```python
from build123d import *

# Parameters (mm, degrees)
BOSS_EXTRUDE1_DEPTH = 4
SKETCH2_R           = 1.6
CUT_EXTRUDE1_DEPTH  = 80.797158741
CUT_EXTRUDE2_DEPTH  = 2
CUT_EXTRUDE3_DEPTH  = 1.5
SKETCH5_R           = 4
BOSS_EXTRUDE3_DEPTH = 2
SKETCH6_R           = 1.5
CUT_EXTRUDE4_DEPTH  = 80.797158741
FILLET1_R           = 3


with BuildPart() as part:
    # Sketch1 → Boss-Extrude1 (new body)
    with BuildSketch(Plane(origin=(0, 0, 0), x_dir=(1, 0, 0), z_dir=(0, 1, 0))):
        Polygon((-12.5, 0), (12.5, 0), (23.338026386, 1.062677778), (36.065948447, -11.665244283), (35.003270669, -22.503270669), (35.003270669, -47.503270669), (36.065948447, -58.341297055), (23.338026386, -71.069219116), (12.5, -70.006541338), (-12.5, -70.006541338), (-23.338026386, -71.069219116), (-36.065948447, -58.341297055), (-35.003270669, -47.503270669), (-35.003270669, -22.503270669), (-36.065948447, -11.665244283), (-23.338026386, 1.062677778), align=None)
    extrude(amount=BOSS_EXTRUDE1_DEPTH)

    # Sketch2 → Cut-Extrude1 (cut, through all)
    with BuildSketch(Plane(origin=(0, 4, 0), x_dir=(1, 0, 0), z_dir=(0, 1, 0))):
        with Locations(Location((22.63, -3.893270669, 0), (0, 0, 270))):
            Circle(SKETCH2_R)
        with Locations(Location((31.11, -12.373270669, 0), (0, 0, 270))):
            Circle(SKETCH2_R)
        with Locations(Location((-31.11, -12.373270669, 0), (0, 0, 90))):
            Circle(SKETCH2_R)
        with Locations(Location((-22.63, -3.893270669, 0), (0, 0, 90))):
            Circle(SKETCH2_R)
        with Locations(Location((31.11, -57.633270669, 0), (0, 0, 90))):
            Circle(SKETCH2_R)
        with Locations(Location((22.63, -66.113270669, 0), (0, 0, 90))):
            Circle(SKETCH2_R)
        with Locations(Location((-22.63, -66.113270669, 0), (0, 0, 270))):
            Circle(SKETCH2_R)
        with Locations(Location((-31.11, -57.633270669, 0), (0, 0, 270))):
            Circle(SKETCH2_R)
    extrude(amount=-CUT_EXTRUDE1_DEPTH, mode=Mode.SUBTRACT)

    # Sketch3 → Cut-Extrude2 (cut)
    with BuildSketch(Plane(origin=(0, 4, 0), x_dir=(1, 0, 0), z_dir=(0, 1, 0))):
        Polygon((-17.672782103, -6), (17.672782103, -6), (29.003270669, -17.330488566), (29.003270669, -52.676052772), (17.672782103, -64.006541338), (-17.672782103, -64.006541338), (-29.003270669, -52.676052772), (-29.003270669, -17.330488566), align=None)
    extrude(amount=-CUT_EXTRUDE2_DEPTH, mode=Mode.SUBTRACT)

    # Sketch4 → Cut-Extrude3 (cut)
    with BuildSketch(Plane(origin=(0, 2, 0), x_dir=(1, 0, 0), z_dir=(0, 1, 0))):
        with BuildLine():
            Line((-4.595346553, -50.006541338), (4.595346553, -50.006541338))
            ThreePointArc((4.595346553, -50.006541338), (5.867462624, -50.289609115), (6.899515315, -51.085394202))
            Line((6.899515315, -51.085394202), (13.569676517, -59.085394202))
            ThreePointArc((13.569676517, -59.085394202), (13.982439977, -62.278657408), (11.265507754, -64.006541338))
            Line((11.265507754, -64.006541338), (-11.265507754, -64.006541338))
            ThreePointArc((-11.265507754, -64.006541338), (-13.982439977, -62.278657408), (-13.569676517, -59.085394202))
            Line((-13.569676517, -59.085394202), (-6.899515315, -51.085394202))
            ThreePointArc((-6.899515315, -51.085394202), (-5.867462624, -50.289609115), (-4.595346553, -50.006541338))
        make_face()
        with BuildLine():
            Line((-24.082123534, -48.572947186), (-16.082123534, -41.902785984))
            ThreePointArc((-16.082123534, -41.902785984), (-15.286338446, -40.870733292), (-15.003270669, -39.598617222))
            Line((-15.003270669, -39.598617222), (-15.003270669, -30.407924116))
            ThreePointArc((-15.003270669, -30.407924116), (-15.286338446, -29.135808045), (-16.082123534, -28.103755354))
            Line((-16.082123534, -28.103755354), (-24.082123534, -21.433594152))
            ThreePointArc((-24.082123534, -21.433594152), (-27.27538674, -21.020830692), (-29.003270669, -23.737762914))
            Line((-29.003270669, -23.737762914), (-29.003270669, -46.268778423))
            ThreePointArc((-29.003270669, -46.268778423), (-27.27538674, -48.985710646), (-24.082123534, -48.572947186))
        make_face()
        with BuildLine():
            Line((-13.569676517, -10.921147135), (-6.899515315, -18.921147135))
            ThreePointArc((-6.899515315, -18.921147135), (-5.867462624, -19.716932223), (-4.595346553, -20))
            Line((-4.595346553, -20), (4.595346553, -20))
            ThreePointArc((4.595346553, -20), (5.867462624, -19.716932223), (6.899515315, -18.921147135))
            Line((6.899515315, -18.921147135), (13.569676517, -10.921147135))
            ThreePointArc((13.569676517, -10.921147135), (13.982439977, -7.727883929), (11.265507754, -6))
            Line((11.265507754, -6), (-11.265507754, -6))
            ThreePointArc((-11.265507754, -6), (-13.982439977, -7.727883929), (-13.569676517, -10.921147135))
        make_face()
        with BuildLine():
            Line((24.082123534, -21.433594152), (16.082123534, -28.103755354))
            ThreePointArc((16.082123534, -28.103755354), (15.286338446, -29.135808045), (15.003270669, -30.407924116))
            Line((15.003270669, -30.407924116), (15.003270669, -39.598617222))
            ThreePointArc((15.003270669, -39.598617222), (15.286338446, -40.870733292), (16.082123534, -41.902785984))
            Line((16.082123534, -41.902785984), (24.082123534, -48.572947186))
            ThreePointArc((24.082123534, -48.572947186), (27.27538674, -48.985710646), (29.003270669, -46.268778423))
            Line((29.003270669, -46.268778423), (29.003270669, -23.737762914))
            ThreePointArc((29.003270669, -23.737762914), (27.27538674, -21.020830692), (24.082123534, -21.433594152))
        make_face()
    extrude(amount=-CUT_EXTRUDE3_DEPTH, mode=Mode.SUBTRACT)

    # Sketch5 → Boss-Extrude3 (add)
    with BuildSketch(Plane(origin=(0, 2, 0), x_dir=(1, 0, 0), z_dir=(0, 1, 0))):
        with Locations(Location((15.25, -19.753270669, 0), (0, 0, 90))):
            Circle(SKETCH5_R)
        with Locations(Location((-15.25, -19.753270669, 0), (0, 0, 90))):
            Circle(SKETCH5_R)
        with Locations(Location((-15.25, -50.253270669, 0), (0, 0, 90))):
            Circle(SKETCH5_R)
        with Locations(Location((15.25, -50.253270669, 0), (0, 0, 90))):
            Circle(SKETCH5_R)
    extrude(amount=BOSS_EXTRUDE3_DEPTH)

    # Sketch6 → Cut-Extrude4 (cut, through all)
    with BuildSketch(Plane(origin=(0, 4, 0), x_dir=(1, 0, 0), z_dir=(0, 1, 0))):
        with Locations(Location((15.25, -19.753270669, 0), (0, 0, 270))):
            Circle(SKETCH6_R)
        with Locations(Location((15.25, -50.253270669, 0), (0, 0, 270))):
            Circle(SKETCH6_R)
        with Locations(Location((-15.25, -50.253270669, 0), (0, 0, 270))):
            Circle(SKETCH6_R)
        with Locations(Location((-15.25, -19.753270669, 0), (0, 0, 270))):
            Circle(SKETCH6_R)
    extrude(amount=-CUT_EXTRUDE4_DEPTH, mode=Mode.SUBTRACT)

    # Fillet1
    # the kernel refuses this fillet: 3 mm, written as the material it adds along each edge
    with BuildSketch(Plane(origin=(15.25, 2, 19.753270669), x_dir=(0, 0, -1), z_dir=(1, 0, 0))) as fillet1_piece_1:
        with BuildLine():
            CenterArc((6.828427125, 3), FILLET1_R, 199.471220634, 70.528779366)
            Line((4, 2), (3.943431458, 1.98))
            ThreePointArc((3.943431458, 1.98), (3.94, 1), (3.94, 0))
            Line((3.94, 0), (4, -0.06))
            Line((4, -0.06), (6.828427125, -0.06))
            Line((6.828427125, -0.06), (6.828427125, 0))
        make_face()
    revolve(axis=Axis((15.25, 2, 19.753270669), (0, 1, 0)))
    with BuildSketch(Plane(origin=(-15.25, 2, 19.753270669), x_dir=(0, 0, -1), z_dir=(1, 0, 0))) as fillet1_piece_2:
        with BuildLine():
            CenterArc((6.828427125, 3), FILLET1_R, 199.471220634, 70.528779366)
            Line((4, 2), (3.943431458, 1.98))
            ThreePointArc((3.943431458, 1.98), (3.94, 1), (3.94, 0))
            Line((3.94, 0), (4, -0.06))
            Line((4, -0.06), (6.828427125, -0.06))
            Line((6.828427125, -0.06), (6.828427125, 0))
        make_face()
    revolve(axis=Axis((-15.25, 2, 19.753270669), (0, 1, 0)))
    with BuildSketch(Plane(origin=(-15.25, 2, 50.253270669), x_dir=(0, 0, -1), z_dir=(1, 0, 0))) as fillet1_piece_3:
        with BuildLine():
            CenterArc((6.828427125, 3), FILLET1_R, 199.471220634, 70.528779366)
            Line((4, 2), (3.943431458, 1.98))
            ThreePointArc((3.943431458, 1.98), (3.94, 1), (3.94, 0))
            Line((3.94, 0), (4, -0.06))
            Line((4, -0.06), (6.828427125, -0.06))
            Line((6.828427125, -0.06), (6.828427125, 0))
        make_face()
    revolve(axis=Axis((-15.25, 2, 50.253270669), (0, 1, 0)))
    with BuildSketch(Plane(origin=(15.25, 2, 50.253270669), x_dir=(0, 0, -1), z_dir=(1, 0, 0))) as fillet1_piece_4:
        with BuildLine():
            CenterArc((6.828427125, 3), FILLET1_R, 199.471220634, 70.528779366)
            Line((4, 2), (3.943431458, 1.98))
            ThreePointArc((3.943431458, 1.98), (3.94, 1), (3.94, 0))
            Line((3.94, 0), (4, -0.06))
            Line((4, -0.06), (6.828427125, -0.06))
            Line((6.828427125, -0.06), (6.828427125, 0))
        make_face()
    revolve(axis=Axis((15.25, 2, 50.253270669), (0, 1, 0)))


solid = part.part
```
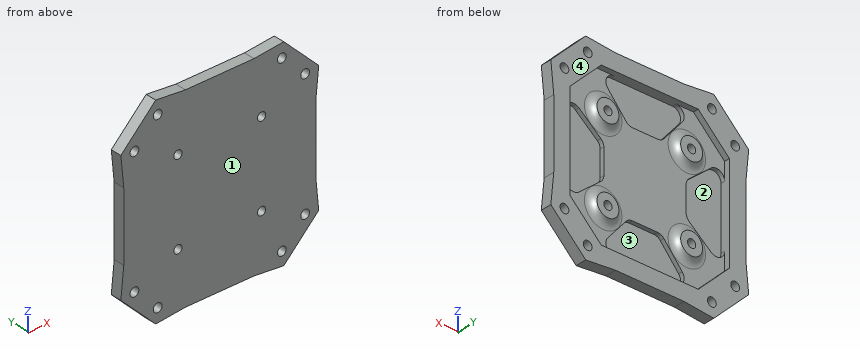
Work out the finished part from the listing and answer in its coordinate system (mm). Face numbers are marked on the shaded views. A direction names the side the tool comes from. Coordinates: 2 decimals unless noted, no trailing zeros. Loops run counter-clockwise (first coordinate to the right, second up) from the corner with the lowest first, then second, coordinate; pieces in that order, holes last. Notation, with made-up numbers: (-28.5, 12.25) - (-5.5, 12.25) arc R16 ccw to (-5.5, 23.25) - close; hole circle Ø2 at (75.25, 57.25). An arc over 180 degrees is marked (long way). Use a Markdown table: item, result.
Item 1: Find section C-C, the plane y = 2.7. State how many separate pieces and enclosed holes the cut face has, and give its area (3 significant figures).
Evaluation:
| item | result |
|---|---|
| separate pieces | 5 |
| enclosed holes | 13 |
| area | 1,830 mm2 |
Item 2: Given pin 1 Ø2.5 at (x, z) = (22.63, 3.89) entering from -Y; pin 2 Ø11 at (x, z) = (-19.5, 39.5) entering from +Y; pin 3 Ø11 at (x, z) = (0.5, 14) entering from +Y; pin 4 Ø1.5 at (x, z) = (21, 56.5) entering from -Y, each flat-ended and moving along its own axis, determine where each tip first touches the part or whether it passes through.
Evaluation:
| item | result |
|---|---|
| pin 1 | passes through |
| pin 2 | stops at y = 2.1 |
| pin 3 | stops at y = 0.5 |
| pin 4 | stops at y = 0 |
Item 3: For the marked faces 1 and 2, determine the directions among +Z, -Z, +X, -X, +Y, -Y from which every point of the face is accessible in a straight line to the end or side of a thin tool.
Evaluation:
| item | result |
|---|---|
| face 1 | +Z, -Z, +X, -X, -Y |
| face 2 | +Y |
Item 4: Consider probe 1 along X at (y, z) = (1.3, 36); probe 2 along Z at (x, y) = (23.5, 2.45); probe 3 along Z at (x, y) = (6, 2.65). Determine where each line is inside the solid, lowest interval first. Write a range as from..to.
Evaluation:
| item | result |
|---|---|
| probe 1 | x = -35..-29, -15..15, 29..35 |
| probe 2 | z = -0.9..2.55, 5.24..11.83, 58.18..64.77, 67.46..70.91 |
| probe 3 | z = 0..6, 64.01..70.01 |
Item 5: Find section A-A, the plane x = -31.11. Determine the outline of the cut face in (y, z), and give its area (3 significant figures).
Evaluation:
| item | result |
|---|---|
| outline | (0, 6.71) - (4, 6.71) - (4, 10.77) - (0, 10.77) - close; (0, 13.97) - (4, 13.97) - (4, 56.03) - (0, 56.03) - close; (0, 59.23) - (4, 59.23) - (4, 63.3) - (0, 63.3) - close |
| area | 201 mm2 |
Item 6: The mould has two halves that part along Z. Classify the marked faces 3 and 4: +Z half, -Z half, draft (parallel to the pull), parting line (faces both ways), or undercut.
Evaluation:
| item | result |
|---|---|
| face 3 | undercut |
| face 4 | draft |
Item 7: Find section B-B, the plane z = 66. Determine the outline of the cut face in (x, y), and give its area (3 significant figures).
Evaluation:
| item | result |
|---|---|
| outline | (-28.41, 0) - (-24.23, 0) - (-24.23, 4) - (-28.41, 4) - close; (-21.03, 0) - (21.03, 0) - (21.03, 4) - (-21.03, 4) - close; (24.23, 0) - (28.41, 0) - (28.41, 4) - (24.23, 4) - close |
| area | 202 mm2 |
